Read the model definition and answer for the solid it produces. Units are mm, in the model's axes. A direction names the side the tool comes from. Coordinates: 2 decimals unless noted, no trailing zeros. Write each loop counter-clockwise with the first axis right and the second up, starting at its lowest first coordinate (ties: lowest second). Pieces come first, ordered by that corner, then holes. Notation, with made-up numbers: (-29.75, -37.75) -> (9.25, -37.75) arc R14 cw to (9.25, -32.75) -> close; hole circle Ø11 at (41.5, -29). An arc over 180 degrees is marked (long way). Use CSV: the item, a comma, the result in double quotes.
from build123d import *

# Parameters (mm, degrees)
BOSS_EXTRUDE1_DEPTH = 28
CUT_EXTRUDE1_DEPTH  = 90.677477663
SKETCH5_R           = 6.35
CUT_EXTRUDE2_DEPTH  = 4.572
SKETCH8_R           = 6.35
SKETCH8_R_2         = 4.318
BOSS_EXTRUDE4_DEPTH = 6.858
CUT_EXTRUDE6_START  = -2.54
CUT_EXTRUDE6_DEPTH  = 91.021953984
SKETCH14_W          = 51.838761269
SKETCH14_H          = 46.114624518
CUT_EXTRUDE7_DEPTH  = 83.190253836


with BuildPart() as part:
    # Sketch2 → Boss-Extrude1 (new body)
    with BuildSketch(Plane(origin=(0, 0, 0), x_dir=(1, 0, 0), z_dir=(0, 1, 0))):
        with BuildLine():
            Line((-38.1, -65.991135768), (0, 0))
            Line((0, 0), (0, -76.2))
            ThreePointArc((0, -76.2), (-19.722011237, -73.603547963), (-38.1, -65.991135768))
        make_face()
    boss_extrude1 = extrude(amount=BOSS_EXTRUDE1_DEPTH)

    # Sketch4 → Cut-Extrude1 (cut, symmetric)
    with BuildSketch(Plane(origin=(0, 28, 0), x_dir=(1, 0, 0), z_dir=(0, 1, 0))):
        Polygon((-19.722011237, -73.603547963), (-19.722011237, -45.603553163), (19.722011237, -45.603553163), (19.722011237, -73.603547963), (19.722011237, -89.083413221), (-19.722011237, -89.083413221), align=None)
    cut_extrude1 = extrude(amount=CUT_EXTRUDE1_DEPTH, both=True, mode=Mode.SUBTRACT)

    # Sketch5 → Cut-Extrude2 (cut)
    with BuildSketch(Plane(origin=(-19.722011237, 0, 0), x_dir=(0, 0, -1), z_dir=(1, 0, 0))):
        with Locations((-64.683550563, 14)):
            Circle(SKETCH5_R)
    cut_extrude2 = extrude(amount=-CUT_EXTRUDE2_DEPTH, mode=Mode.SUBTRACT)

    # Sketch8 → Boss-Extrude4 (add)
    with BuildSketch(Plane(origin=(-19.722011237, 0, 0), x_dir=(0, 0, -1), z_dir=(1, 0, 0))):
        with Locations((-64.683550563, 14)):
            Circle(SKETCH8_R)
        with Locations((-64.683550563, 14)):
            Circle(SKETCH8_R_2, mode=Mode.SUBTRACT)
    boss_extrude4 = extrude(amount=-BOSS_EXTRUDE4_DEPTH)

    # Sketch13 → Cut-Extrude6 (cut)
    with BuildSketch(Plane(origin=(0, 0, 0), x_dir=(1, 0, 0), z_dir=(0, 1, 0)).offset(CUT_EXTRUDE6_START)):
        Polygon((-23.532011237, -79.497992122), (-59.753612954, -79.497992122), (-59.753612954, -51.700018712), (-33.00752403, -46.22932884), (-23.532011237, -36.276651464), (-23.532011237, -51.700018712), align=None)
        with BuildLine():
            Line((-6.646719096, -17.852832416), (-17.283715983, -36.276651464))
            Line((-17.283715983, -36.276651464), (-10.73360519, -40.058359694))
            Line((-10.73360519, -40.058359694), (-3.170188732, -40.058359694))
            Line((-3.170188732, -40.058359694), (-3.170188732, -18.78436593))
            ThreePointArc((-3.170188732, -18.78436593), (-4.930502865, -18.400886976), (-6.646719096, -17.852832416))
        make_face()
    cut_extrude6 = extrude(amount=CUT_EXTRUDE6_DEPTH, mode=Mode.SUBTRACT)

    # Sketch14 → Cut-Extrude7 (cut, symmetric)
    with BuildSketch(Plane(origin=(0, 28, 0), x_dir=(1, 0, 0), z_dir=(0, 1, 0))):
        with Locations((2.387369397, -17.701326807)):
            Rectangle(SKETCH14_W, SKETCH14_H)
    cut_extrude7 = extrude(amount=CUT_EXTRUDE7_DEPTH, both=True, mode=Mode.SUBTRACT)

    # Mirror2: Boss-Extrude1, Cut-Extrude1, Cut-Extrude2, Boss-Extrude4, Cut-Extrude6, Cut-Extrude7 across plane
    add(boss_extrude1.mirror(Plane(origin=(0, 28, 0), x_dir=(0, 0, 1), z_dir=(-1, 0, 0))))
    add(cut_extrude1.mirror(Plane(origin=(0, 28, 0), x_dir=(0, 0, 1), z_dir=(-1, 0, 0))), mode=Mode.SUBTRACT)
    add(cut_extrude2.mirror(Plane(origin=(0, 28, 0), x_dir=(0, 0, 1), z_dir=(-1, 0, 0))), mode=Mode.SUBTRACT)
    add(boss_extrude4.mirror(Plane(origin=(0, 28, 0), x_dir=(0, 0, 1), z_dir=(-1, 0, 0))))
    add(cut_extrude6.mirror(Plane(origin=(0, 28, 0), x_dir=(0, 0, 1), z_dir=(-1, 0, 0))), mode=Mode.SUBTRACT)
    add(cut_extrude7.mirror(Plane(origin=(0, 28, 0), x_dir=(0, 0, 1), z_dir=(-1, 0, 0))), mode=Mode.SUBTRACT)


solid = part.part
1. A cutting plane is placed at B-B (y = 14). Give the vertices of the cut face in (x, z), and give its area (3 significant figures).
Solutions:
outline,"(-23.53, 40.76) -> (23.53, 40.76) -> (23.53, 60.37) -> (19.72, 60.37) -> (19.72, 45.6) -> (-19.72, 45.6) -> (-19.72, 60.37) -> (-23.53, 60.37) -> close; (-23.53, 69) -> (-19.72, 69) -> (-19.72, 73.6) arc R76.2 ccw to (-23.53, 72.48) -> close; (19.72, 69) -> (23.53, 69) -> (23.53, 72.48) arc R76.2 ccw to (19.72, 73.6) -> close"
area,"371 mm^2"
2. A tool of negligible diameter and unlimited length cuts with its end or side. For faces 1 (the flat face through (19.722, 14, 60)), 2 (the cylindrical face through (21.61, 13.8, 73.07)), from which of +Z, -Z, +X, -X, +Y, -Y can it reach the whole face along a straight path? Write none if from no direction.
Solutions:
face 1,"+Z, +Y, -Y"
face 2,"+Z, +X, +Y, -Y"
3. Each of these flat-tipped pins is pushed along its axis until it touches: pin 1 Ø7 at (y, z) = (14, 64.68) entering from +X; pin 2 Ø10 at (y, z) = (14, 64.68) entering from -X. Where does it stop, or does it pass through?
Solutions:
pin 1,"passes through"
pin 2,"stops at x = -23.53"
4. A cutting plane is placed at D-D (x = -15). Give the vertices of the cut face in (y, z).
Solutions:
outline,"(0, 40.76) -> (28, 40.76) -> (28, 45.6) -> (0, 45.6) -> close"
5. Find the intervals of material crossed by line 1 along X through (y, z) = (14, 47); line 2 along Z through (x, y) = (-9, 5); line 3 along Z through (x, y) = (22.3, 14), in increasing order.
Solutions:
line 1,"x = -23.53 to -19.72, 19.72 to 23.53"
line 2,"z = 40.76 to 45.6"
line 3,"z = 40.76 to 60.37, 69 to 72.86"
6. A cutting plane is placed at A-A (z = 55). Give the vertices of the cut face in (x, y), and give its area (3 significant figures).
Solutions:
outline,"(-23.53, 0) -> (-19.72, 0) -> (-19.72, 28) -> (-23.53, 28) -> close; (19.72, 0) -> (23.53, 0) -> (23.53, 28) -> (19.72, 28) -> close"
area,"213 mm^2"
7. A cutting plane is placed at C-C (z = 61.5). Give the vertices of the cut face in (x, y), and give its area (3 significant figures).
Solutions:
outline,"(-23.53, 0) -> (-19.72, 0) -> (-19.72, 11.08) -> (-23.53, 11.08) -> close; (-23.53, 16.92) -> (-19.72, 16.92) -> (-19.72, 28) -> (-23.53, 28) -> close; (19.72, 0) -> (23.53, 0) -> (23.53, 11.08) -> (19.72, 11.08) -> close; (19.72, 16.92) -> (23.53, 16.92) -> (23.53, 28) -> (19.72, 28) -> close"
area,"169 mm^2"
8. For a pull along Y with two mould halves and no side action, classify faces 3 (the flat face through (0, 28, 45)), 4 (the cylindrical face through (-21.6, 15.297, 60.565)), 5 (the flat face through (0, 14, 45.604)) as pulls with the +Y half, pulls with the -Y half, needs draft (parallel to the pull), parting line crosses it, or undercut.
Solutions:
face 3,"pulls with the +Y half"
face 4,"undercut"
face 5,"needs draft"
